Autodesk Inventor part; units mm, degrees
ref_plane "YZ Plane" through (0, 0, 0) normal (1, 0, 0) x (0, 1, 0)
ref_plane "XZ Plane" through (0, 0, 0) normal (0, 1, 0) x (-1, 0, 0)
ref_plane "XY Plane" through (0, 0, 0) normal (0, 0, 1) x (1, 0, 0)
sketch "Sketch1" plane through (0, 0, 0) normal (0, 1, 0) x (-1, 0, 0)
  line L0 (0, 0) -> (177.8, 0)
  line L1 (177.8, 0) -> (177.8, -142.24)
  line L2 (177.8, -142.24) -> (0, -142.24)
  line L3 (0, -142.24) -> (0, 0)
  line L4 (177.8, 0) -> (88.9, 0)
  line L5 (88.9, 0) -> (114.3, 0)
  line L6 (114.3, 0) -> (63.5, 0)
  line L7 (63.5, 0) -> (63.5, -8.255)
  line L8 (63.5, -8.255) -> (63.5, -20.955)
  line L9 (63.5, -20.955) -> (114.3, -20.955)
  line L10 (114.3, -20.955) -> (114.3, -8.255)
  point P0 (116.227, -12.0777)
  dimension "d0" = 177.8
  dimension "d1" = 142.24
  dimension "d2" = 25.4
  dimension "d3" = 50.8
  dimension "d4" = 8.255
  dimension "d5" = 12.7
  dimension "d6" = 50.8
extrude "Extrusion1" add sketch "Sketch1" along normal blind 6.35
hole "Hole1" at (-63.5, 0, -8.255) at (-63.5, 0, -20.955) at (-114.3, 0, -20.955) at (-114.3, 0, -8.255) direction (0, 1, 0) diameter 6.7564 end through all
sketch "Sketch2" plane through (0, 6.35, 0) normal (0, 1, 0) x (1, 0, 0)
  line L0 (-177.8, 142.24) -> (-177.8, 0)
  line L1 (-177.8, 142.24) -> (-171.45, 142.24)
  line L2 (-171.45, 142.24) -> (-171.45, 139.7)
  line L3 (-171.45, 139.7) -> (-177.8, 139.7)
  line L4 (-177.8, 139.7) -> (-177.8, 142.24)
  line L5 (-171.45, 139.7) -> (-98.6688, 139.7)
  line L6 (-98.6688, 139.7) -> (-98.6688, 24.6405)
  line L7 (-98.6688, 24.6405) -> (-171.45, 24.6405)
  line L8 (-171.45, 24.6405) -> (-171.45, 139.7)
  line L9 (0, 142.24) -> (-177.8, 142.24)
  line L10 (0, 142.24) -> (-6.35, 142.24)
  line L11 (-6.35, 142.24) -> (-6.35, 139.7)
  line L12 (-6.35, 139.7) -> (0, 139.7)
  line L13 (0, 139.7) -> (0, 142.24)
  line L14 (-6.35, 139.7) -> (-79.121, 139.7)
  line L15 (-79.121, 139.7) -> (-79.121, 24.6405)
  line L16 (-79.121, 24.6405) -> (-6.35, 24.6405)
  line L17 (-6.35, 24.6405) -> (-6.35, 139.7)
  point P0 (0, 0)
  dimension "d16" = 6.35
  dimension "d17" = 2.54
  dimension "d18" = 72.7812
  dimension "d19" = 115.0595
  dimension "d20" = 6.35
  dimension "d21" = 72.771
  dimension "d22" = 115.0595
extrude "Extrusion2" cut sketch "Sketch2" against normal blind 6.35 contours L17 L16 L15 L14 | L5 L6 L7 L8
sketch "Sketch3" plane through (0, 6.35, 0) normal (0, 1, 0) x (1, 0, 0)
  line L0 (-98.6688, 139.7) -> (-171.45, 139.7)
  line L1 (-98.6688, 139.7) -> (-96.1288, 139.7)
  line L2 (-96.1288, 139.7) -> (-96.1288, 24.6405)
  line L3 (-96.1288, 24.6405) -> (-98.6688, 24.6405)
  line L4 (-98.6688, 24.6405) -> (-98.6688, 139.7)
  line L5 (-79.121, 24.6405) -> (-79.121, 139.7)
  line L6 (-79.121, 24.6405) -> (-81.661, 24.6405)
  line L7 (-81.661, 24.6405) -> (-81.661, 139.7)
  line L8 (-81.661, 139.7) -> (-79.121, 139.7)
  line L9 (-79.121, 139.7) -> (-79.121, 24.6405)
  line L10 (-96.1288, 139.7) -> (-93.5888, 139.7)
  line L11 (-93.5888, 139.7) -> (-93.5888, 24.6405)
  line L12 (-93.5888, 24.6405) -> (-96.1288, 24.6405)
  line L13 (-96.1288, 24.6405) -> (-96.1288, 139.7)
  line L14 (-81.661, 24.6405) -> (-84.201, 24.6405)
  line L15 (-84.201, 24.6405) -> (-84.201, 139.7)
  line L16 (-84.201, 139.7) -> (-81.661, 139.7)
  line L17 (-81.661, 139.7) -> (-81.661, 24.6405)
  line L18 (-93.5888, 139.7) -> (-84.201, 139.7)
  line L19 (-84.201, 139.7) -> (-84.201, 24.6405)
  line L20 (-84.201, 24.6405) -> (-93.5888, 24.6405)
  line L21 (-93.5888, 24.6405) -> (-93.5888, 139.7)
  point P0 (0, 0)
  dimension "d26" = 2.54
  dimension "d27" = 2.54
  dimension "d30" = 2.54
  dimension "d31" = 2.54
extrude "Extrusion4" add sketch "Sketch3" along normal blind 1.27 contours L10 L11 L12 L2 | L18 L15 L20 L11 | L16 L7 L14 L15
properties part number "USAXS double well plate"
Input: part model. Units: mm. Frame: model coordinates. A direction names the side the tool comes from. Coordinates: 2 decimals unless noted, no trailing zeros. Order: outer loops, then holes, each group sorted by start corner. A loop starts at its lowest first (then second) coordinate and runs counter-clockwise, first axis right, second up. Notation, with made-up numbers: (59, 85.5) - (101, 85.5) arc R20 cw to (101, 89.5) - close; hole circle Ø9 at (43, -20.5). An arc over 180 degrees is marked (long way). Put each result on its own line as item: value.
1. Reachability of faces 5 (the face through (-171.45, 3, -81)), 6 (the face through (-88, 0, -50)) from +Z, -Z, +X, -X, +Y, -Y: full face, straight path, thin tool, end or side. Return the list, or none.
Report:
face 5: +Y, -Y
face 6: +Z, -Z, +X, -X, -Y
2. Cut plane A-A on z = -116.5. Return the cut outline in (x, y), then the cut area to 3 significant figures.
Report:
outline: (-177.8, 0) - (-171.45, 0) - (-171.45, 6.35) - (-177.8, 6.35) - close; (-98.67, 0) - (-79.12, 0) - (-79.12, 6.35) - (-81.66, 6.35) - (-81.66, 7.62) - (-96.13, 7.62) - (-96.13, 6.35) - (-98.67, 6.35) - close; (-6.35, 0) - (0, 0) - (0, 6.35) - (-6.35, 6.35) - close
area: 223 mm2
3. Contact query for flat-ended pins moving along their axis: pin 1 Ø0.6 at (x, y) = (-89, 7) entering from -Z; pin 2 Ø9 at (x, z) = (-114.3, -20.955) entering from +Y; pin 3 Ø0.6 at (y, z) = (7, -78) entering from -X. Output: stop coordinate, or through.
Report:
pin 1: stops at z = -139.7
pin 2: stops at y = 6.35
pin 3: stops at x = -96.13
4. Draft query along Z for faces 1 (the face through (-88, 3, 0)), 2 (the face through (-79.121, 3, -83)), 3 (the face through (-177.8, 3, -70)), 4 (the face through (-135, 3, -24.64)). Return one class per face: pulls with the +Z half, pulls with the -Z half, needs draft (parallel to the pull), parting line crosses it, or undercut.
Report:
face 1: pulls with the +Z half
face 2: undercut
face 3: needs draft
face 4: undercut
5. Line query: line 1 along X through (y, z) = (3.5, -39); line 2 along Z through (x, y) = (-114.3, 2.5); line 3 along Z through (x, y) = (-78, 4). Output: solid intervals per line, ascending.
Report:
line 1: x = -177.8 to -171.45, -98.67 to -79.12, -6.35 to 0
line 2: z = -142.24 to -139.7, -24.64 to -24.33, -17.58 to -11.63, -4.88 to 0
line 3: z = -142.24 to -139.7, -24.64 to 0
6. Cut plane B-B on x = -73. Return the cut outline in (y, z).
Report:
outline: (0, -142.24) - (6.35, -142.24) - (6.35, -139.7) - (0, -139.7) - close; (0, -24.64) - (6.35, -24.64) - (6.35, 0) - (0, 0) - close
7. Cut plane C-C on y = 5. State how many separate pieces and enclosed holes the cut face has, then the cut area to 3 significant figures.
Report:
separate pieces: 1
enclosed holes: 6
area: 8,400 mm2
